Study the drawing (mm; zero at the part's minimum x, y, z) and answer. A direction names the side the tool comes from. Give positions to 0.01 mm unless a question says otherwise; leave off trailing zeros. Write each loop counter-clockwise with the first axis right and the second up, starting at its lowest first coordinate (ties: lowest second). Pieces come first, ordered by that corner, then holes. Notation, with made-up numbers: (-34, 79) -> (6, 79) arc R5 cw to (6, 86) -> close; hole circle Ø8 at (20, 68). An arc over 180 degrees is marked (long way). Put each result on its own line as item: value. Start each with the question number.
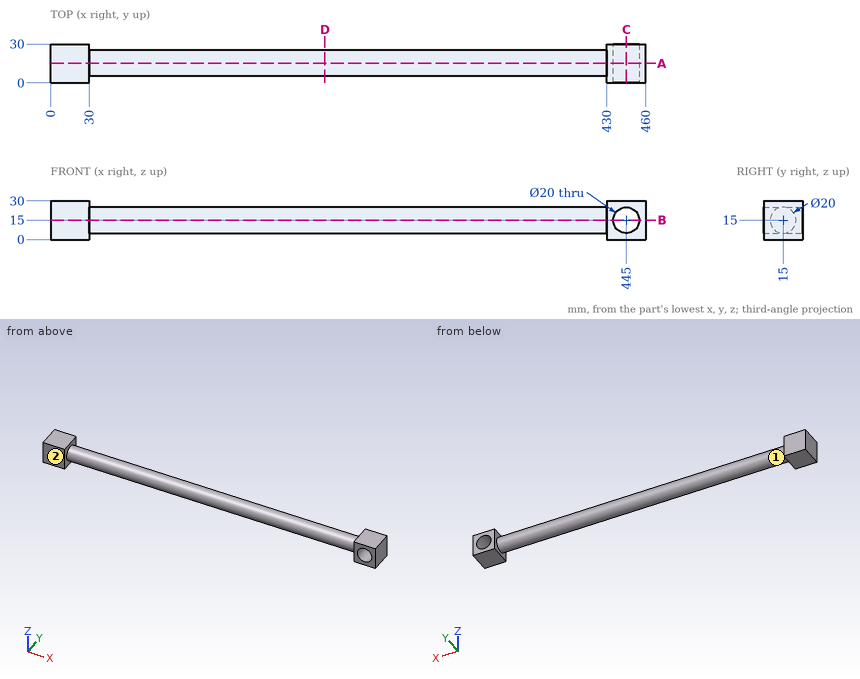
1) Straight lines are drawn through the part: line 1 (Z direction, x = 445, y = 9.75); line 2 (X direction, y = 7, z = 26.25); line 3 (X direction, y = 18.75, z = 15). For each, find the intervals that lie inside material, in ascending order. Write a range as [from, to].
2) Each of these flat-tipped pins is pushed along its axis until it touches: pin 1 Ø1.5 at (x, z) = (349.5, 24) entering from -Y; pin 2 Ø6 at (x, z) = (194, 23.5) entering from -Y; pin 3 Ø12 at (x, z) = (368, 5.5) entering from -Y; pin 4 Ø4 at (y, z) = (19.5, 16) entering from -X. Where does it stop, or does it pass through?
3) A cutting plane is placed at A-A on y = 15. Give the vertices of the cut face in (x, z), and give its area (3 significant figures).
4) For the marked faces 1 and 2, determine the directions among +Z, -Z, +X, -X, +Y, -Y from which every point of the face is accessible in a straight line to the end or side of a thin tool.
5) A cutting plane is placed at C-C on x = 445. Give the vertices of the cut face in (y, z).
6) A cutting plane is placed at B-B on z = 15. Give the vertices of the cut face in (x, y), and give its area (3 significant figures).
7) A cutting plane is placed at D-D on x = 212. Give the vertices of the cut face in (y, z).
Results found:
1. line 1: z = [0, 5], [25, 30]
1. line 2: x = [0, 30], [430, 460]
1. line 3: x = [0, 435], [455, 460]
2. pin 1: stops at y = 9.35
2. pin 2: stops at y = 6.65
2. pin 3: stops at y = 5.63
2. pin 4: stops at x = 0
3. outline: (0, 0) -> (30, 0) -> (30, 5) -> (430, 5) -> (430, 0) -> (460, 0) -> (460, 30) -> (430, 30) -> (430, 25) -> (30, 25) -> (30, 30) -> (0, 30) -> close; hole circle Ø20 at (445, 15)
3. area: 9,490 mm²
4. face 1: none
4. face 2: +Z, -Z, +X, -X, -Y
5. outline: (0, 0) -> (30, 0) -> (30, 5) -> (0, 5) -> close; (0, 25) -> (30, 25) -> (30, 30) -> (0, 30) -> close
6. outline: (0, 0) -> (30, 0) -> (30, 5) -> (430, 5) -> (430, 0) -> (435, 0) -> (435, 30) -> (430, 30) -> (430, 25) -> (30, 25) -> (30, 30) -> (0, 30) -> close; (455, 0) -> (460, 0) -> (460, 30) -> (455, 30) -> close
6. area: 9,200 mm²
7. outline: circle Ø20 at (15, 15)
